Answer from the drawing. Dimensions are ordinates in mm from the lowest x, y and z of the part. Give positions to 0.01 mm unless a question says otherwise; leave off trailing zeros. Loops run counter-clockwise (first coordinate to the right, second up) from the corner with the lowest first, then second, coordinate; pieces in that order, holes last. Notation, with made-up numbers: (-28, 73.5) -> (6, 73.5) arc R31 ccw to (6, 109.5) -> close; hole circle Ø1 at (-36, 80). An arc over 180 degrees is marked (long way). Return JSON: item names as keys, results as strings. Group by question number.
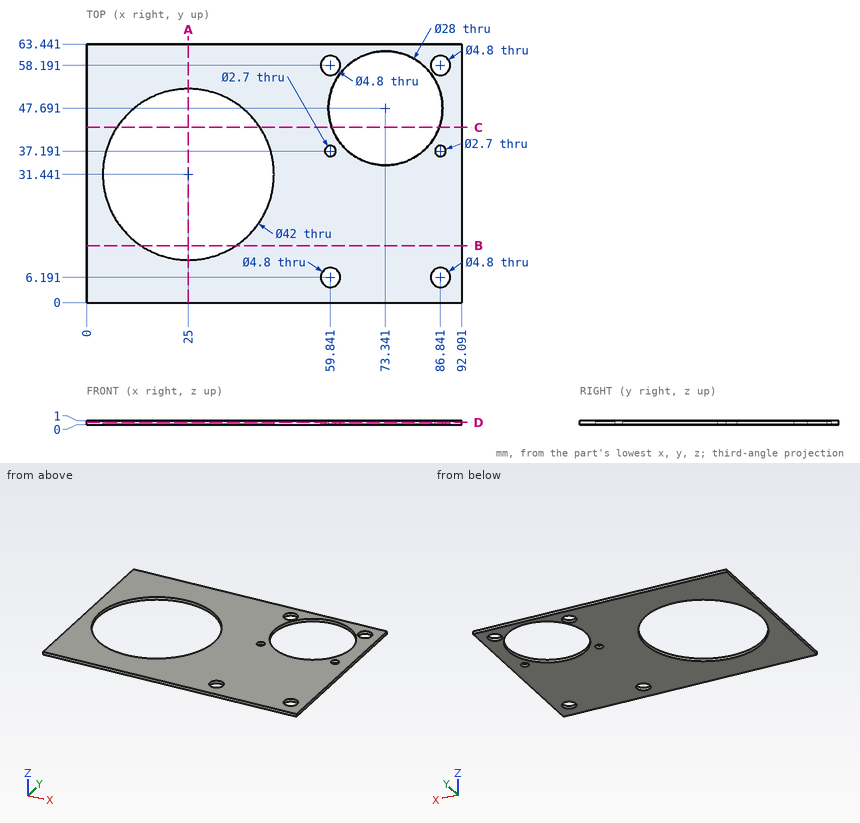
1. Section B-B on y = 14 is taken. Determine the outline of the cut face in (x, z).
2. Section A-A on x = 25 is taken. Determine the outline of the cut face in (y, z).
3. Section C-C on y = 43 is taken. Determine the outline of the cut face in (x, z).
4. A flat-ended cylindrical pin translates along its axis: pin 1 Ø2 at (x, y) = (86.84, 37.19) entering from -Z. Find the tip coordinate at first contact, or state that the pin passes through.
5. Section D-D on z = 0.55 is taken. State how many separate pieces and enclosed holes the cut face has, then the cut area to 3 significant figures.
6. Straight lines are drawn through the part: line 1 (X direction, y = 43.5, z = 0.4); line 2 (Y direction, x = 59, z = 0.3) (1 decimal); line 3 (X direction, y = 49, z = 0.95). For each, find the intervals that lie inside material, in ascending order. Write a range as from..to.
Completed:
{
 "1": {"outline": "(0, 0) -> (13.3, 0) -> (13.3, 1) -> (0, 1) -> close; (36.7, 0) -> (92.09, 0) -> (92.09, 1) -> (36.7, 1) -> close"},
 "2": {"outline": "(0, 0) -> (10.44, 0) -> (10.44, 1) -> (0, 1) -> close; (52.44, 0) -> (63.44, 0) -> (63.44, 1) -> (52.44, 1) -> close"},
 "3": {"outline": "(0, 0) -> (7.47, 0) -> (7.47, 1) -> (0, 1) -> close; (42.53, 0) -> (60.15, 0) -> (60.15, 1) -> (42.53, 1) -> close; (86.53, 0) -> (92.09, 0) -> (92.09, 1) -> (86.53, 1) -> close"},
 "4": {"pin 1": "passes through"},
 "5": {"separate pieces": "1", "enclosed holes": "8", "area": "3,760 mm²"},
 "6": {"line 1": "x = 0..7.81, 42.19..59.98, 86.7..92.09", "line 2": "y = 0..3.9, 8.4..36.1, 38.2..55.9, 60.4..63.4", "line 3": "x = 0..13.48, 36.52..59.4, 87.28..92.09"}
}
